```python
from build123d import *

# Parameters (mm, degrees)
BOSS_EXTRUDE1_DEPTH = 20
FILLET1_R           = 20
CUT_EXTRUDE1_REACH  = 66.376
SKETCH2_R           = 1.75
CUT_EXTRUDE2_REACH  = 66.376


with BuildPart() as part:
    # Sketch1 → Boss-Extrude1 (new, symmetric)
    with BuildSketch(Plane.XY):
        Polygon((0, 44.5), (0, 0), (44.5, 0), (44.5, 2.5), (2.5, 2.5), (2.5, 44.5), align=None)
    extrude(amount=BOSS_EXTRUDE1_DEPTH, both=True)

    # Fillet1
    fillet1_edges = [part.edges().sort_by_distance(p)[0] for p in [
        (1.25, 44.5, -20),
        (1.25, 44.5, 20),
    ]]
    fillet(fillet1_edges, radius=FILLET1_R - 0.0001)  # a hair under: the kernel refuses the full size

    # Sketch2 → Cut-Extrude1 (cut, up to next)
    with BuildSketch(Plane(origin=(2.5, 0, 0), x_dir=(0, 0, -1), z_dir=(1, 0, 0)), mode=Mode.PRIVATE) as cut_extrude1_sk1:
        with Locations(Location((9.899494937, 14.600505063, 0), (0, 0, 90))):
            Circle(SKETCH2_R)
    cut_extrude1_tool1 = extrude(cut_extrude1_sk1.sketch, amount=-CUT_EXTRUDE1_REACH, mode=Mode.PRIVATE) & part.part
    # Sketch2 → Cut-Extrude1 (cut, up to next)
    with BuildSketch(Plane(origin=(2.5, 0, 0), x_dir=(0, 0, -1), z_dir=(1, 0, 0)), mode=Mode.PRIVATE) as cut_extrude1_sk2:
        with Locations(Location((-9.899494937, 14.600505063, 0), (0, 0, 90))):
            Circle(SKETCH2_R)
    cut_extrude1_tool2 = extrude(cut_extrude1_sk2.sketch, amount=-CUT_EXTRUDE1_REACH, mode=Mode.PRIVATE) & part.part
    # Sketch2 → Cut-Extrude1 (cut, up to next)
    with BuildSketch(Plane(origin=(2.5, 0, 0), x_dir=(0, 0, -1), z_dir=(1, 0, 0)), mode=Mode.PRIVATE) as cut_extrude1_sk3:
        with Locations(Location((-9.899494937, 34.399494937, 0), (0, 0, 90))):
            Circle(SKETCH2_R)
    cut_extrude1_tool3 = extrude(cut_extrude1_sk3.sketch, amount=-CUT_EXTRUDE1_REACH, mode=Mode.PRIVATE) & part.part
    # Sketch2 → Cut-Extrude1 (cut, up to next)
    with BuildSketch(Plane(origin=(2.5, 0, 0), x_dir=(0, 0, -1), z_dir=(1, 0, 0)), mode=Mode.PRIVATE) as cut_extrude1_sk4:
        with Locations(Location((9.899494937, 34.399494937, 0), (0, 0, 90))):
            Circle(SKETCH2_R)
    cut_extrude1_tool4 = extrude(cut_extrude1_sk4.sketch, amount=-CUT_EXTRUDE1_REACH, mode=Mode.PRIVATE) & part.part
    # Sketch2 → Cut-Extrude1 (cut, up to next)
    with BuildSketch(Plane(origin=(2.5, 0, 0), x_dir=(0, 0, -1), z_dir=(1, 0, 0)), mode=Mode.PRIVATE) as cut_extrude1_sk5:
        with BuildLine():
            Line((10.25, 29.136809248), (10.25, 19.863190752))
            ThreePointArc((10.25, 19.863190752), (0, 13.25), (-10.25, 19.863190752))
            Line((-10.25, 19.863190752), (-10.25, 29.136809248))
            ThreePointArc((-10.25, 29.136809248), (0, 35.75), (10.25, 29.136809248))
        make_face()
    cut_extrude1_tool5 = extrude(cut_extrude1_sk5.sketch, amount=-CUT_EXTRUDE1_REACH, mode=Mode.PRIVATE) & part.part
    add(cut_extrude1_tool1.solids().sort_by_distance((2.5, 14.600505, -9.899495))[0], mode=Mode.SUBTRACT)
    add(cut_extrude1_tool2.solids().sort_by_distance((2.5, 14.600505, 9.899495))[0], mode=Mode.SUBTRACT)
    add(cut_extrude1_tool3.solids().sort_by_distance((2.5, 34.399495, 9.899495))[0], mode=Mode.SUBTRACT)
    add(cut_extrude1_tool4.solids().sort_by_distance((2.5, 34.399495, -9.899495))[0], mode=Mode.SUBTRACT)
    add(cut_extrude1_tool5.solids().sort_by_distance((2.5, 24.5, 0))[0], mode=Mode.SUBTRACT)

    # Sketch3 → Cut-Extrude2 (cut, up to next)
    with BuildSketch(Plane(origin=(0, 2.5, 0), x_dir=(1, 0, 0), z_dir=(0, 1, 0)), mode=Mode.PRIVATE) as cut_extrude2_sk1:
        with BuildLine():
            Line((13.25, -10), (13.25, -15))
            ThreePointArc((13.25, -15), (11.5, -16.75), (9.75, -15))
            Line((9.75, -15), (9.75, -10))
            ThreePointArc((9.75, -10), (11.5, -8.25), (13.25, -10))
        make_face()
    cut_extrude2_tool1 = extrude(cut_extrude2_sk1.sketch, amount=-CUT_EXTRUDE2_REACH, mode=Mode.PRIVATE) & part.part
    # Sketch3 → Cut-Extrude2 (cut, up to next)
    with BuildSketch(Plane(origin=(0, 2.5, 0), x_dir=(1, 0, 0), z_dir=(0, 1, 0)), mode=Mode.PRIVATE) as cut_extrude2_sk2:
        with BuildLine():
            Line((41.25, -10), (41.25, -15))
            ThreePointArc((41.25, -15), (39.5, -16.75), (37.75, -15))
            Line((37.75, -15), (37.75, -10))
            ThreePointArc((37.75, -10), (39.5, -8.25), (41.25, -10))
        make_face()
    cut_extrude2_tool2 = extrude(cut_extrude2_sk2.sketch, amount=-CUT_EXTRUDE2_REACH, mode=Mode.PRIVATE) & part.part
    # Sketch3 → Cut-Extrude2 (cut, up to next)
    with BuildSketch(Plane(origin=(0, 2.5, 0), x_dir=(1, 0, 0), z_dir=(0, 1, 0)), mode=Mode.PRIVATE) as cut_extrude2_sk3:
        with BuildLine():
            Line((13.25, 15), (13.25, 10))
            ThreePointArc((13.25, 10), (11.5, 8.25), (9.75, 10))
            Line((9.75, 10), (9.75, 15))
            ThreePointArc((9.75, 15), (11.5, 16.75), (13.25, 15))
        make_face()
    cut_extrude2_tool3 = extrude(cut_extrude2_sk3.sketch, amount=-CUT_EXTRUDE2_REACH, mode=Mode.PRIVATE) & part.part
    # Sketch3 → Cut-Extrude2 (cut, up to next)
    with BuildSketch(Plane(origin=(0, 2.5, 0), x_dir=(1, 0, 0), z_dir=(0, 1, 0)), mode=Mode.PRIVATE) as cut_extrude2_sk4:
        with BuildLine():
            Line((41.25, 15), (41.25, 10))
            ThreePointArc((41.25, 10), (39.5, 8.25), (37.75, 10))
            Line((37.75, 10), (37.75, 15))
            ThreePointArc((37.75, 15), (39.5, 16.75), (41.25, 15))
        make_face()
    cut_extrude2_tool4 = extrude(cut_extrude2_sk4.sketch, amount=-CUT_EXTRUDE2_REACH, mode=Mode.PRIVATE) & part.part
    add(cut_extrude2_tool1.solids().sort_by_distance((11.5, 2.5, 12.5))[0], mode=Mode.SUBTRACT)
    add(cut_extrude2_tool2.solids().sort_by_distance((39.5, 2.5, 12.5))[0], mode=Mode.SUBTRACT)
    add(cut_extrude2_tool3.solids().sort_by_distance((11.5, 2.5, -12.5))[0], mode=Mode.SUBTRACT)
    add(cut_extrude2_tool4.solids().sort_by_distance((39.5, 2.5, -12.5))[0], mode=Mode.SUBTRACT)


solid = part.part
```
CAD build for the part. Positions are in the model's coordinates, mm. A direction names the side the tool comes from. Round coordinates to 2 decimals unless told otherwise and drop trailing zeros. Write each loop counter-clockwise with the first axis right and the second up, starting at its lowest first coordinate (ties: lowest second). Pieces come first, ordered by that corner, then holes. Notation, with made-up numbers: (88, 35) - (103, 35) arc R32 cw to (103, 71) - close; hole circle Ø4 at (-3.75, 18.5). An arc over 180 degrees is marked (long way). Return JSON: item names as keys, results as strings. Group by question number.
Item 1: Band-saw the part on B-B on x = 39.5. List the corners of the cut face in (y, z), plus the area to 3 significant figures.
Item 2: Probe probe 1 along Y at (x, z) = (34, 9.5). List the from-to ranges inside material, lowest first.
Item 3: Band-saw the part on C-C on z = 9. List the corners of the cut face in (x, y), plus the area to 3 significant figures.
Item 4: 3-axis set-ups, long thin cutter, end or side, ignore diameter. For faces 1 (the face through (9.75, 1, 13)), 2 (the face through (1.27, 13.25, -0.18)), 3 (the face through (14, 2, -20)): which of +Z, -Z, +X, -X, +Y, -Y reach the whole face in a straight line?
Item 5: Band-saw the part on A-A on y = 22. List the corners of the cut face in (x, z), plus the area to 4 significant figures.
Item 6: Flat gauge pins, fed straight in: pin 1 Ø1.2 at (y, z) = (1.5, -12) entering from -X; pin 2 Ø2 at (x, y) = (1.5, 26) entering from -Z; pin 3 Ø4 at (x, z) = (31, 1.5) entering from +Y. Where does each tip first touch, or does it go through?
Item 7: Mould opens along Y. For faces 4 (the face through (24, 2.5, 0)), 5 (the face through (44.5, 1, 0)), 6 (the face through (1.27, 35.75, 0.18)) say: +Y half, -Y half, draft (parallel to the pull), parting line (faces both ways), or undercut.
Item 8: Band-saw the part on D-D on z = 3. List the corners of the cut face in (x, y), plus the area to 3 significant figures.
Resolved:
{
 "1": {"outline": "(0, -20) - (2.5, -20) - (2.5, -16.75) - (0, -16.75) - close; (0, -8.25) - (2.5, -8.25) - (2.5, 8.25) - (0, 8.25) - close; (0, 16.75) - (2.5, 16.75) - (2.5, 20) - (0, 20) - close", "area": "57.5 mm²"},
 "2": {"probe 1": "y = 0 to 2.5"},
 "3": {"outline": "(0, 0) - (10.06, 0) - (10.06, 2.5) - (2.5, 2.5) - (2.5, 13.1) - (0, 13.1) - close; (0, 16.1) - (2.5, 16.1) - (2.5, 17.75) - (0, 17.75) - close; (0, 31.25) - (2.5, 31.25) - (2.5, 32.9) - (0, 32.9) - close; (0, 35.9) - (2.5, 35.9) - (2.5, 42.36) - (0, 42.36) - close; (12.94, 0) - (38.06, 0) - (38.06, 2.5) - (12.94, 2.5) - close; (40.94, 0) - (44.5, 0) - (44.5, 2.5) - (40.94, 2.5) - close", "area": "148 mm²"},
 "4": {"face 1": "+Y, -Y", "face 2": "+X, -X", "face 3": "-Z, +X, -X, +Y, -Y"},
 "5": {"outline": "(0, -20) - (2.5, -20) - (2.5, -10.25) - (0, -10.25) - close; (0, 10.25) - (2.5, 10.25) - (2.5, 20) - (0, 20) - close", "area": "48.75 mm²"},
 "6": {"pin 1": "stops at x = 0", "pin 2": "stops at z = -19.99", "pin 3": "stops at y = 2.5"},
 "7": {"face 4": "+Y half", "face 5": "draft", "face 6": "undercut"},
 "8": {"outline": "(0, 0) - (44.5, 0) - (44.5, 2.5) - (2.5, 2.5) - (2.5, 13.66) - (0, 13.66) - close; (0, 35.34) - (2.5, 35.34) - (2.5, 44.27) - (0, 44.27) - close", "area": "161 mm²"}
}
